Read the model definition and answer for the solid it produces. Units are mm, in the model's axes. A direction names the side the tool comes from. Coordinates: 2 decimals unless noted, no trailing zeros. Order: outer loops, then holes, each group sorted by start corner. A loop starts at its lowest first (then second) coordinate and runs counter-clockwise, first axis right, second up. Notation, with made-up numbers: M -10.5,-28 L 1.5,-28 A15 cw 1.5,-13 Z; hole C 75.5,47.5 d10. An arc over 180 degrees is marked long. Put each result on its own line as item: value.
from build123d import *

# Parameters (mm, degrees)
SKETCH_1_W             = 48
SKETCH_1_H             = 125
EXTRUDE_403_DEPTH      = 2
SKETCH_2_W             = 9
SKETCH_2_H             = 35
CUT_EXTRUDE_733_DEPTH  = 67.979474468
SKETCH_3_W             = 7
SKETCH_3_H             = 55
EXTRUDE_1088_DEPTH     = 7
SKETCH_4_W             = 30
SKETCH_4_H             = 3
EXTRUDE_1396_DEPTH     = 7
SKETCH_5_R             = 1.65
CUT_EXTRUDE_1704_DEPTH = 68.551831951
SKETCH_7_R             = 3
CUT_EXTRUDE_2019_DEPTH = 4
CHAMFER_1_SIZE         = 1.5
FILLET_1_R             = 1.5
FILLET_2_R             = 2
FILLET_3_R             = 3.5


# Some blends are built 0.0001 mm under size
with BuildPart() as part:
    # Эскиз1 → Extrude 403 (new body)
    with BuildSketch(Plane(origin=(0, 0, 0), x_dir=(1, 0, 0), z_dir=(0, 1, 0))):
        Rectangle(SKETCH_1_W, SKETCH_1_H)
    extrude(amount=EXTRUDE_403_DEPTH)

    # Эскиз2 → Cut-Extrude 733 (cut, through all)
    with BuildSketch(Plane(origin=(0, 2, 0), x_dir=(1, 0, 0), z_dir=(0, 1, 0))):
        with Locations((-19.5, 45)):
            Rectangle(SKETCH_2_W, SKETCH_2_H)
        with Locations((19.5, 45)):
            Rectangle(SKETCH_2_W, SKETCH_2_H)
        with Locations((19.5, -45)):
            Rectangle(SKETCH_2_W, SKETCH_2_H)
        with Locations((-19.5, -45)):
            Rectangle(SKETCH_2_W, SKETCH_2_H)
    extrude(amount=-CUT_EXTRUDE_733_DEPTH, mode=Mode.SUBTRACT)

    # Эскиз3 → Extrude 1088 (add)
    with BuildSketch(Plane(origin=(0, 2, 0), x_dir=(1, 0, 0), z_dir=(0, 1, 0))):
        with Locations((-20.5, 0)):
            Rectangle(SKETCH_3_W, SKETCH_3_H)
        with Locations((20.5, 0)):
            Rectangle(SKETCH_3_W, SKETCH_3_H)
    extrude(amount=EXTRUDE_1088_DEPTH)

    # Эскиз4 → Extrude 1396 (add)
    with BuildSketch(Plane(origin=(0, 2, 0), x_dir=(1, 0, 0), z_dir=(0, 1, 0))):
        with Locations((0, 61)):
            Rectangle(SKETCH_4_W, SKETCH_4_H)
        with Locations((0, -61)):
            Rectangle(SKETCH_4_W, SKETCH_4_H)
    extrude(amount=EXTRUDE_1396_DEPTH)

    # Эскиз5 → Cut-Extrude 1704 (cut, through all)
    with BuildSketch(Plane(origin=(0, 9, 0), x_dir=(1, 0, 0), z_dir=(0, 1, 0))):
        with Locations(Location((-20.5, 22.5, 0), (0, 0, 270))):
            Circle(SKETCH_5_R)
        with Locations(Location((-20.5, -22.5, 0), (0, 0, 270))):
            Circle(SKETCH_5_R)
        with Locations(Location((20.5, -22.5, 0), (0, 0, 270))):
            Circle(SKETCH_5_R)
        with Locations(Location((20.5, 22.5, 0), (0, 0, 270))):
            Circle(SKETCH_5_R)
    extrude(amount=-CUT_EXTRUDE_1704_DEPTH, mode=Mode.SUBTRACT)

    # Эскиз7 → Cut-Extrude 2019 (cut)
    with BuildSketch(Plane.XZ):
        with Locations(Location((-20.5, 22.5, 0), (0, 0, 270))):
            Circle(SKETCH_7_R)
        with Locations(Location((-20.5, -22.5, 0), (0, 0, 270))):
            Circle(SKETCH_7_R)
        with Locations(Location((20.5, 22.5, 0), (0, 0, 270))):
            Circle(SKETCH_7_R)
        with Locations(Location((20.5, -22.5, 0), (0, 0, 270))):
            Circle(SKETCH_7_R)
    extrude(amount=-CUT_EXTRUDE_2019_DEPTH, mode=Mode.SUBTRACT)

    # Фаска1
    # the kernel refuses this chamfer: 1.5 mm, written as the material it takes off along each edge
    with BuildSketch(Plane(origin=(-20.5, 4, 22.5), x_dir=(0, 0, 1), z_dir=(-1, 0, 0))) as chamfer_1_piece_1_section:
        Polygon((1.65 + CHAMFER_1_SIZE, 0), (1.65, CHAMFER_1_SIZE), (1.65, 0), align=None)
    chamfer_1_piece_1 = revolve(axis=Axis((-20.5, 4, 22.5), (0, 1, 0)), mode=Mode.PRIVATE)
    chamfer_1_piece_1 = chamfer_1_piece_1 & Plane(origin=(-20.5, 4.828305934, 22.5), x_dir=(0, 0, -1), z_dir=(0, -1, 0)) * Cylinder(3, 13, mode=Mode.PRIVATE)
    add(chamfer_1_piece_1, mode=Mode.SUBTRACT)
    with BuildSketch(Plane(origin=(-20.5, 4, -22.5), x_dir=(0, 0, 1), z_dir=(-1, 0, 0))) as chamfer_1_piece_2_section:
        Polygon((1.65 + CHAMFER_1_SIZE, 0), (1.65, CHAMFER_1_SIZE), (1.65, 0), align=None)
    chamfer_1_piece_2 = revolve(axis=Axis((-20.5, 4, -22.5), (0, 1, 0)), mode=Mode.PRIVATE)
    chamfer_1_piece_2 = chamfer_1_piece_2 & Plane(origin=(-20.5, 4.828305934, -22.5), x_dir=(0, 0, -1), z_dir=(0, -1, 0)) * Cylinder(3, 13, mode=Mode.PRIVATE)
    add(chamfer_1_piece_2, mode=Mode.SUBTRACT)
    with BuildSketch(Plane(origin=(20.5, 4, -22.5), x_dir=(0, 0, 1), z_dir=(-1, 0, 0))) as chamfer_1_piece_3_section:
        Polygon((1.65 + CHAMFER_1_SIZE, 0), (1.65, CHAMFER_1_SIZE), (1.65, 0), align=None)
    chamfer_1_piece_3 = revolve(axis=Axis((20.5, 4, -22.5), (0, 1, 0)), mode=Mode.PRIVATE)
    chamfer_1_piece_3 = chamfer_1_piece_3 & Plane(origin=(20.5, 4.828305934, -22.5), x_dir=(0, 0, -1), z_dir=(0, -1, 0)) * Cylinder(3, 13, mode=Mode.PRIVATE)
    add(chamfer_1_piece_3, mode=Mode.SUBTRACT)
    with BuildSketch(Plane(origin=(20.5, 4, 22.5), x_dir=(0, 0, 1), z_dir=(-1, 0, 0))) as chamfer_1_piece_4_section:
        Polygon((1.65 + CHAMFER_1_SIZE, 0), (1.65, CHAMFER_1_SIZE), (1.65, 0), align=None)
    chamfer_1_piece_4 = revolve(axis=Axis((20.5, 4, 22.5), (0, 1, 0)), mode=Mode.PRIVATE)
    chamfer_1_piece_4 = chamfer_1_piece_4 & Plane(origin=(20.5, 4.828305934, 22.5), x_dir=(0, 0, -1), z_dir=(0, -1, 0)) * Cylinder(3, 13, mode=Mode.PRIVATE)
    add(chamfer_1_piece_4, mode=Mode.SUBTRACT)

    # Скругление1
    fillet_1_edges = [part.edges().sort_by_distance(p)[0] for p in [
        (-15, 5.5, 59.5),
        (-15, 4.5, 62.5),
        (15, 4.5, 62.5),
        (15, 5.5, 59.5),
        (15, 4.5, -62.5),
        (15, 5.5, -59.5),
        (-15, 5.5, -59.5),
        (-15, 4.5, -62.5),
    ]]
    fillet(fillet_1_edges, radius=FILLET_1_R - 0.0001)  # a hair under: the kernel refuses the full size

    # Скругление2
    fillet_2_edges = [part.edges().sort_by_distance(p)[0] for p in [
        (15, 1, -27.5),
        (-15, 1, -27.5),
        (-15, 1, 27.5),
        (15, 1, 27.5),
    ]]
    fillet(fillet_2_edges, radius=FILLET_2_R)

    # Скругление3
    fillet_3_edges = [part.edges().sort_by_distance(p)[0] for p in [
        (-17, 5.5, 27.5),
        (-24, 4.5, 27.5),
        (-24, 4.5, -27.5),
        (-17, 5.5, -27.5),
        (24, 4.5, -27.5),
        (17, 5.5, -27.5),
        (17, 5.5, 27.5),
        (24, 4.5, 27.5),
    ]]
    fillet(fillet_3_edges, radius=FILLET_3_R - 0.0001)  # a hair under: the kernel refuses the full size


solid = part.part
Q1. For a pull along Z with two mould halves and no side action, classify faces 5 (the face through (23, 4.44, -26.45)), 6 (the face through (0, 0, -1)), 7 (the face through (21.615, 7.274, 21.284)), 8 (the face through (18.05, 5.55, 26.5)) as +Z half, -Z half, draft (parallel to the pull), parting line (faces both ways), or undercut.
Answers below:
face 5: -Z half
face 6: draft
face 7: undercut
face 8: +Z half
Q2. Find section D-D on z = 7. Write down the section's boundary in (x, y).
Answers below:
outline: M -24,0 L 24,0 L 24,9 L 17,9 L 17,2 L -17,2 L -17,9 L -24,9 Z
Q3. Consider line 1 along Z through (x, y) = (20.5, 2.35); line 2 along X through (y, z) = (8.25, -22.5); line 3 along X through (y, z) = (3.1, 22.5). Determine where each line is inside the solid, lowest interval first.
Answers below:
line 1: z = -27.5 to -25.5, -19.5 to 19.5, 25.5 to 27.5
line 2: x = -24 to -22.15, -18.85 to -17, 17 to 18.85, 22.15 to 24
line 3: x = -24 to -23.5, -17.5 to -17, 17 to 17.5, 23.5 to 24
Q4. Find section A-A on z = -22.5. Write down the section's boundary in (x, y), plus the area to 3 significant figures.
Answers below:
outline: M -24,0 L -23.5,0 L -23.5,4.15 L -22.15,5.5 L -22.15,9 L -24,9 Z; M -18.85,5.5 L -17.5,4.15 L -17.5,0 L 17.5,0 L 17.5,4.15 L 18.85,5.5 L 18.85,9 L 17,9 L 17,2 L -17,2 L -17,9 L -18.85,9 Z; M 22.15,5.5 L 23.5,4.15 L 23.5,0 L 24,0 L 24,9 L 22.15,9 Z
area: 109 mm^2
Q5. Given pin 1 (4.5 mm diameter, centred on y = 3, z = -38.5, fed in from -X); pin 2 (3.5 mm diameter, centred on x = 20.5, z = -22.5, fed in from -Y); pin 3 (1.8 mm diameter, centred on x = 18.5, y = 3.5, fed in from +Z); pin 4 (3 mm diameter, centred on x = -20.5, z = 22.5, fed in from -Y), each flat-ended and moving along its own axis, determine where each tip first touches the part or whether it passes through.
Answers below:
pin 1: stops at x = -15
pin 2: stops at y = 5.4
pin 3: stops at z = 27.32
pin 4: passes through
Q6. Find section B-B on y = 7.75. Give the number of separate pieces and of enclosed holes in the cut face, plus the area to 3 significant figures.
Answers below:
separate pieces: 4
enclosed holes: 4
area: 891 mm^2
Q7. A tool of negligible diameter and unlimited length cuts with its end or side. For faces 1 (the face through (-18.05, 5.55, -26.5)), 2 (the face through (18.7, 2, -20.1)), 3 (the face through (0, 2, -1)), 4 (the face through (19, 1, 27.5)), from which of +Z, -Z, +X, -X, +Y, -Y can it reach the whole face along a straight path? Write none if from no direction.
Answers below:
face 1: -Z, +Y
face 2: -Y
face 3: +Y
face 4: +Z, +X, +Y, -Y
Q8. Find section C-C on x = -6. Write down the section's boundary in (y, z), plus the area to 3 significant figures.
Answers below:
outline: M 0,-62.5 L 9,-62.5 L 9,-59.5 L 2,-59.5 L 2,59.5 L 9,59.5 L 9,62.5 L 0,62.5 Z
area: 292 mm^2
